Geometry: final body of the model. Coordinates: model frame, mm. A direction names the side the tool comes from. Round coordinates to 2 decimals unless told otherwise and drop trailing zeros. Loops run counter-clockwise (first coordinate to the right, second up) from the corner with the lowest first, then second, coordinate; pieces in that order, holes last. Notation, with made-up numbers: (-35.75, -22) - (-6.75, -22) arc R20 cw to (-6.75, -1) - close; hole circle Ø6 at (14.25, -36). An arc over 180 degrees is marked (long way). Answer as a JSON object with one key per item and string values. Group by question number.
Item 1: Draft query along X for faces 1 (the face through (-23.1, 6.27, -9.86)), 2 (the face through (0.4, 7.125, -10.5)), 3 (the face through (21, 0, -10)), 4 (the face through (-13.79, -5.6, -4.97)). Return one class per face: released by +X, released by -X, zero draft, split by the parting line, or undercut.
Item 2: Reachability of faces 5 (the face through (0, -4.125, -12)), 6 (the face through (-31.145, -6.223, 2.465)), 7 (the face through (23.145, 6.223, -9.86)), 8 (the face through (18.21, -5.6, -4.97)), 9 (the face through (-23.145, -6.223, -9.86)) from +Z, -Z, +X, -X, +Y, -Y: full face, straight path, thin tool, end or side. Return the list, or none.
Item 3: Section B-B (x = -28). Return the cut outline in (y, z) (3 decimals), plus the area to 4 significant figures.
Item 4: Section C-C (z = -12.25). Return the cut outline in (x, y) (3 decimals), plus the area to 3 significant figures.
Item 5: First-contact query: pin 1 (6.5 mm diameter, centred on y = 0.5, z = -12, fed in from +X); pin 2 (9.5 mm diameter, centred on x = 0, z = -7, fed in from +Y) (3 decimals); pin 3 (2.5 mm diameter, centred on y = 1.5, z = -11.5, fed in from -X); pin 4 (5.5 mm diameter, centred on x = 28, y = 2.5, fed in from -Z). Flat tips, straight axial feed; report the tip coordinate or a pass-through.
Item 6: Section A-A (y = 0). Return the cut outline in (x, z).
Item 7: Section D-D (x = 8). Return the cut outline in (y, z) (3 decimals), plus the area to 3 significant figures.
Item 8: Line query: line 1 (Z direction, x = 8, y = -5.8); line 2 (Y direction, x = 3, z = -10) (3 decimals); line 3 (X direction, y = -5, z = -4.5). Output: solid intervals per line, ascending.
```python
from build123d import *

# Parameters (mm, degrees)
F0_W     = 42
F0_H     = 8.25
F1_DEPTH = 5
F2_DEPTH = 20
F3_R     = 3
F4_DEPTH = 25
F5_D     = 3


with BuildPart() as f1:
    # F0 (on Top) → F1 (new body)
    with BuildSketch(Plane.XY):
        with BuildLine():
            ThreePointArc((-24, 4.125), (-23.12132, 6.24632), (-21, 7.125))
            Line((-21, 7.125), (-29, 7.125))
            ThreePointArc((-29, 7.125), (-31.12132, 6.24632), (-32, 4.125))
            Line((-32, 4.125), (-32, -4.125))
            ThreePointArc((-32, -4.125), (-31.12132, -6.24632), (-29, -7.125))
            Line((-29, -7.125), (-21, -7.125))
            ThreePointArc((-21, -7.125), (-23.12132, -6.24632), (-24, -4.125))
            Line((-24, -4.125), (-24, 4.125))
        make_face()
        with BuildLine():
            ThreePointArc((24, 4.125), (23.12132, 6.24632), (21, 7.125))
            Line((21, 7.125), (-21, 7.125))
            ThreePointArc((-21, 7.125), (-23.12132, 6.24632), (-24, 4.125))
            Line((-24, 4.125), (-24, -4.125))
            ThreePointArc((-24, -4.125), (-23.12132, -6.24632), (-21, -7.125))
            Line((-21, -7.125), (21, -7.125))
            ThreePointArc((21, -7.125), (23.12132, -6.24632), (24, -4.125))
            Line((24, -4.125), (24, 4.125))
        make_face()
        Rectangle(F0_W, F0_H, mode=Mode.SUBTRACT)
        with BuildLine():
            Line((29, 7.125), (21, 7.125))
            ThreePointArc((21, 7.125), (23.12132, 6.24632), (24, 4.125))
            Line((24, 4.125), (24, -4.125))
            ThreePointArc((24, -4.125), (23.12132, -6.24632), (21, -7.125))
            Line((21, -7.125), (29, -7.125))
            ThreePointArc((29, -7.125), (31.12132, -6.24632), (32, -4.125))
            Line((32, -4.125), (32, 4.125))
            ThreePointArc((32, 4.125), (31.12132, 6.24632), (29, 7.125))
        make_face()
        Rectangle(F0_W, F0_H)
    extrude(amount=F1_DEPTH)

    # F0 (on Top) → F2 (join)
    with BuildSketch(Plane.XY):
        with BuildLine():
            ThreePointArc((24, 4.125), (23.12132, 6.24632), (21, 7.125))
            Line((21, 7.125), (-21, 7.125))
            ThreePointArc((-21, 7.125), (-23.12132, 6.24632), (-24, 4.125))
            Line((-24, 4.125), (-24, -4.125))
            ThreePointArc((-24, -4.125), (-23.12132, -6.24632), (-21, -7.125))
            Line((-21, -7.125), (21, -7.125))
            ThreePointArc((21, -7.125), (23.12132, -6.24632), (24, -4.125))
            Line((24, -4.125), (24, 4.125))
        make_face()
        Rectangle(F0_W, F0_H, mode=Mode.SUBTRACT)
    extrude(amount=-F2_DEPTH)

    # F3 (on face) → F4 (cut)
    with BuildSketch(Plane(origin=(0, 7.125, 0), x_dir=(-1, 0, 0), z_dir=(0, 1, 0))):
        with Locations((-16, -7)):
            Circle(F3_R)
        with Locations((-8, -7)):
            Circle(F3_R)
        with Locations((0, -7)):
            Circle(F3_R)
        with Locations((8, -7)):
            Circle(F3_R)
        with Locations((16, -7)):
            Circle(F3_R)
    extrude(amount=-F4_DEPTH, mode=Mode.SUBTRACT)

    # F5 (through all)
    with Locations(Plane(origin=(0, 0, 0), x_dir=(1, 0, 0), z_dir=(0, 0, -1))):
        with Locations((28, 0), (-28, 0)):
            Hole(F5_D / 2)


solid = f1.part
```
Values:
{
 "1": {"face 1": "released by -X", "face 2": "zero draft", "face 3": "undercut", "face 4": "undercut"},
 "2": {"face 5": "-Z", "face 6": "+Z, -Z, -X, -Y", "face 7": "-Z, +X, +Y", "face 8": "+Y, -Y", "face 9": "-Z, -X, -Y"},
 "3": {"outline": "(-7.125, 0) - (-1.5, 0) - (-1.5, 5) - (-7.125, 5) - close; (1.5, 0) - (7.125, 0) - (7.125, 5) - (1.5, 5) - close", "area": "56.25 mm^2"},
 "4": {"outline": "(-24, -4.125) arc R3 ccw to (-21, -7.125) - (21, -7.125) arc R3 ccw to (24, -4.125) - (24, 4.125) arc R3 ccw to (21, 7.125) - (-21, 7.125) arc R3 ccw to (-24, 4.125) - close; hole (-21, -4.125) - (21, -4.125) - (21, 4.125) - (-21, 4.125) - close", "area": "330 mm^2"},
 "5": {"pin 1": "stops at x = 24", "pin 2": "stops at y = 7.125", "pin 3": "stops at x = -24", "pin 4": "stops at z = 0"},
 "6": {"outline": "(-32, 0) - (-29.5, 0) - (-29.5, 5) - (-32, 5) - close; (-26.5, 0) - (-24, 0) - (-24, -20) - (-21, -20) - (-21, 0) - (21, 0) - (21, -20) - (24, -20) - (24, 0) - (26.5, 0) - (26.5, 5) - (-26.5, 5) - close; (29.5, 0) - (32, 0) - (32, 5) - (29.5, 5) - close"},
 "7": {"outline": "(-7.125, -20) - (-4.125, -20) - (-4.125, -10) - (-7.125, -10) - close; (-7.125, -4) - (-4.125, -4) - (-4.125, 0) - (4.125, 0) - (4.125, -4) - (7.125, -4) - (7.125, 5) - (-7.125, 5) - close; (4.125, -20) - (7.125, -20) - (7.125, -10) - (4.125, -10) - close", "area": "155 mm^2"},
 "8": {"line 1": "z = -20 to -10, -4 to 5", "line 2": "y = -7.125 to -4.125, 4.125 to 7.125", "line 3": "x = -23.87 to -17.66, -14.34 to -9.66, -6.34 to -1.66, 1.66 to 6.34, 9.66 to 14.34, 17.66 to 23.87"}
}
